```python
from build123d import *

# Parameters (mm, degrees)
SKETCH040_W     = 41
SKETCH040_H     = 36
SKETCH040_R     = 1.5
PAD014_DEPTH    = 22
SKETCH041_R     = 2.75
PAD015_DEPTH    = 7
SKETCH042_W     = 21
SKETCH042_H     = 9
PAD016_DEPTH    = 20
SKETCH043_R     = 1.5
PAD017_DEPTH    = 10
POCKET016_DEPTH = 1


with BuildPart() as part:
    # Sketch040 → Pad014 (new body)
    with BuildSketch(Plane.XZ):
        with Locations((-2.5, 0)):
            Rectangle(SKETCH040_W, SKETCH040_H)
        with Locations((15.25, 15.25)):
            Circle(SKETCH040_R, mode=Mode.SUBTRACT)
        with Locations((15.25, -15.25)):
            Circle(SKETCH040_R, mode=Mode.SUBTRACT)
        with Locations((-15.25, -15.25)):
            Circle(SKETCH040_R, mode=Mode.SUBTRACT)
        with Locations((-15.25, 15.25)):
            Circle(SKETCH040_R, mode=Mode.SUBTRACT)
    extrude(amount=PAD014_DEPTH)

    # Sketch041 (on Face9 of Pad014) → Pad015 (join)
    with BuildSketch(Plane(origin=(0, 0, 0), x_dir=(1, 0, 0), z_dir=(0, 1, 0))):
        with Locations((15.25, 15.25)):
            Circle(SKETCH041_R)
        with Locations((15.25, -15.25)):
            Circle(SKETCH041_R)
        with Locations((-15.25, -15.25)):
            Circle(SKETCH041_R)
        with Locations((-15.25, 15.25)):
            Circle(SKETCH041_R)
    extrude(amount=PAD015_DEPTH)

    # Sketch042 (on Face3 of Pad015) → Pad016 (join)
    with BuildSketch(Plane(origin=(18, 0, 0), x_dir=(0, 0, 1), z_dir=(1, 0, 0))):
        with Locations((0, 6.1)):
            Rectangle(SKETCH042_W, SKETCH042_H)
    extrude(amount=PAD016_DEPTH)

    # Sketch043 (on Face2 of Pad016) → Pad017 (join)
    with BuildSketch(Plane(origin=(-23, 0, 0), x_dir=(0, 0, -1), z_dir=(-1, 0, 0))):
        with Locations((-11.5, 2)):
            Circle(SKETCH043_R)
        with Locations((-7.5, 2)):
            Circle(SKETCH043_R)
        with Locations((7.5, 2)):
            Circle(SKETCH043_R)
        with Locations((11.5, 2)):
            Circle(SKETCH043_R)
    extrude(amount=PAD017_DEPTH)

    # Sketch044 (on Face6 of Pad017) → Pocket016 (cut)
    with BuildSketch(Plane.XZ.offset(22)):
        Polygon((-4.106884, -4.719943), (7.24077, 0), (-4.106884, 4.719943), (0, 0), align=None)
    extrude(amount=-POCKET016_DEPTH, mode=Mode.SUBTRACT)


solid = part.part
```
CAD build for the part. Positions are in the model's coordinates, mm. A direction names the side the tool comes from. Coordinates: 2 decimals unless noted, no trailing zeros. Order: outer loops, then holes, each group sorted by start corner. A loop starts at its lowest first (then second) coordinate and runs counter-clockwise, first axis right, second up. Notation, with made-up numbers: (39, 36) -> (73, 36) arc R18 ccw to (73, 55) -> close; hole circle Ø7 at (-36.75, -36.75). An arc over 180 degrees is marked (long way). Use one line per item in the form item = value. Start each with the question number.
1) Band-saw the part on C-C on y = 3.5. Give the cut face in (x, z), then the cut area to 3 significant figures.
2) Band-saw the part on D-D on x = -2. Give the cut face in (y, z), then the cut area to 3 significant figures.
3) Band-saw the part on B-B on z = -7.5. Give the cut face in (x, y), then the cut area to 3 significant figures.
4) Drill centre lines: L1, parallel to Z at x = -15.25, y = -5.25; L2, parallel to Y at x = -21.5, z = -8.5; L3, parallel to X at y = -3.75, z = -10. Where is each one in solid material? Low to high. Write a range as [from, to].
5) Drop flat-ended pins along their axis: pin 1 (10 mm diameter, centred on x = 32, z = -5, fed in from +Y); pin 2 (8 mm diameter, centred on x = 23.5, y = -1, fed in from -Z); pin 3 (1.5 mm diameter, centred on x = -16, z = 0, fed in from +Y). Give the stop position or say it passes through.
6) Tool access for faces 4 (the flat face through (1.646, -21.507, 2.327)), 5 (the cylindrical face through (-28, -2, 13)), 6 (the flat face through (28, -10.6, 0)), 7 (the cylindrical face through (-17.997, 3.451, 15.129)), 8 (the flat face through (28, -1.6, 0)): list every direction of +Z, -Z, +X, -X, +Y, -Y with a clear straight run to the whole face (end or side of a thin tool).
7) Band-saw the part on A-A on y = -5.75. Give the cut face in (x, z), then the cut area to 3 significant figures.
8) Pull direction Z, two halves, no side cores. Call faces 1 (the flat face through (-33, -2, 12)), 2 (the flat face through (-3, -11, -18)), 3 (the cylindrical face through (-15.608, 3.451, -17.977)): +Z half, -Z half, draft (parallel to the pull), parting line (faces both ways), or undercut.
Entries:
q1.outline = circle Ø5.5 at (-15.25, -15.25); circle Ø5.5 at (-15.25, 15.25); circle Ø5.5 at (15.25, -15.25); circle Ø5.5 at (15.25, 15.25)
q1.area = 95.0 mm2
q2.outline = (-22, -18) -> (0, -18) -> (0, 18) -> (-22, 18) -> (-22, 3.84) -> (-21, 3.84) -> (-21, 2.3) -> (-22, 2.3) -> (-22, -2.3) -> (-21, -2.3) -> (-21, -3.84) -> (-22, -3.84) -> close
q2.area = 789 mm2
q3.outline = (-33, -3.5) -> (-23, -3.5) -> (-23, -22) -> (18, -22) -> (18, -10.6) -> (38, -10.6) -> (38, -1.6) -> (18, -1.6) -> (18, 0) -> (-23, 0) -> (-23, -0.5) -> (-33, -0.5) -> close
q3.area = 1,110 mm2
q4.L1 = [-18, -16.75], [-13.75, 13.75], [16.75, 18]
q4.L2 = [-22, 0]
q4.L3 = [-23, 38]
q5.pin_1 = -1.6
q5.pin_2 = -10.5
q5.pin_3 = 0
q6.face_4 = -Y
q6.face_5 = -X
q6.face_6 = +Z, -Z, +X, -Y
q6.face_7 = +Y
q6.face_8 = +Z, -Z, +X, +Y
q7.outline = (-23, -18) -> (18, -18) -> (18, -10.5) -> (38, -10.5) -> (38, 10.5) -> (18, 10.5) -> (18, 18) -> (-23, 18) -> close; hole circle Ø3 at (-15.25, -15.25); hole circle Ø3 at (-15.25, 15.25); hole circle Ø3 at (15.25, -15.25); hole circle Ø3 at (15.25, 15.25)
q7.area = 1,870 mm2
q8.face_1 = draft
q8.face_2 = -Z half
q8.face_3 = undercut
